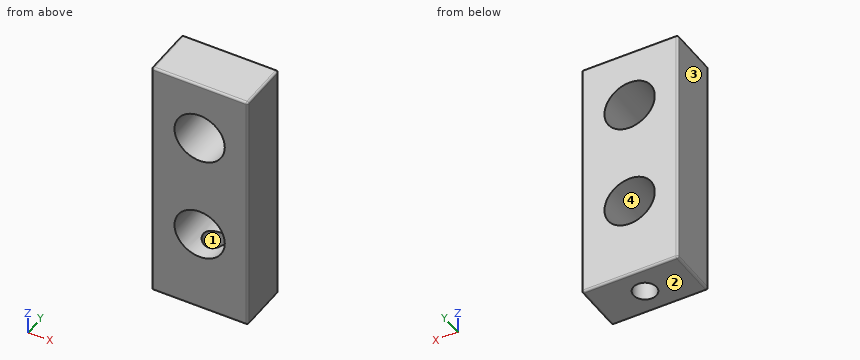
```python
from build123d import *

# Parameters (mm, degrees)
F0_W     = 58.42
F0_H     = 149.86
F0_R     = 15.24
F1_DEPTH = 31.75
F2_R     = 6.985
F3_DEPTH = 46.99
F4_R     = 1.27


with BuildPart() as f1:
    # F0 (on Front) → F1 (new body)
    with BuildSketch(Plane.XZ):
        with Locations((-19.275324, 10.416049)):
            Rectangle(F0_W, F0_H)
        with Locations((-19.275324, -14.983951)):
            Circle(F0_R, mode=Mode.SUBTRACT)
        with Locations((-19.275324, 49.786049)):
            Circle(F0_R, mode=Mode.SUBTRACT)
    extrude(amount=F1_DEPTH)

    # F2 (on face) → F3 (cut)
    with BuildSketch(Plane(origin=(0, 0, -64.513951), x_dir=(1, 0, 0), z_dir=(0, 0, -1))):
        with Locations((-19.275324, 15.875)):
            Circle(F2_R)
    extrude(amount=-F3_DEPTH, mode=Mode.SUBTRACT)

    # F4
    f4_edges = [f1.edges().sort_by_distance(p)[0] for p in [
        (-48.485324, -31.75, 10.416049),
        (9.934676, -31.75, 10.416049),
        (-19.275324, -31.75, -64.513951),
        (-19.275324, -31.75, 85.346049),
        (-48.485324, -15.875, -64.513951),
        (9.934676, -15.875, -64.513951),
        (-48.485324, 0, 10.416049),
        (9.934676, -15.875, 85.346049),
        (9.934676, 0, 10.416049),
        (-19.275324, 0, -64.513951),
        (-19.275324, 0, 85.346049),
        (-48.485324, -15.875, 85.346049),
    ]]
    fillet(f4_edges, radius=F4_R)


solid = f1.part
```
Work out the finished part from the listing and answer in its coordinate system (mm). Face numbers are marked on the shaded views. Give positions to 0.01 mm unless a question says otherwise; leave off trailing zeros. Loops run counter-clockwise (first coordinate to the right, second up) from the corner with the lowest first, then second, coordinate; pieces in that order, holes last. Notation, with made-up numbers: (-15.75, -27.5) - (-3.75, -27.5) arc R31 cw to (-3.75, 6.5) - close; hole circle Ø3 at (80, 51.25). An arc over 180 degrees is marked (long way). Use CSV: the item, a comma, the result in double quotes. Start each with the question number.
(1) Determine the mould class of the marked faces 1, 2, 3 and 4 for opening direction X: released by +X, released by -X, zero draft, split by the parting line, or undercut.
(2) Find section B-B, the plane x = -15.5. Determine the outline of the cut face in (y, z).
(3) Find section D-D, the plane x = -23. Determine the outline of the cut face in (y, z).
(4) Find section C-C, the plane y = -25.5. Determine the outline of the cut face in (x, z), plus the area to 3 significant figures.
(5) Find the intervals of material crossed by L1, parallel to Z at x = -10.5, y = -30; L2, parallel to Z at x = -6, y = -7.5; L3, parallel to X at y = -6.5, z = 63.5, in increasing order.
(6) Find section A-A, the plane z = -20. Determine the outline of the cut face in (x, y), plus the area to 3 significant figures.
Results found:
1,face 1,"undercut"
1,face 2,"zero draft"
1,face 3,"released by -X"
1,face 4,"undercut"
2,outline,"(-31.75, -63.24) arc R1.27 ccw to (-30.48, -64.51) - (-21.75, -64.51) - (-21.75, -29.75) - (-31.75, -29.75) - close; (-31.75, -0.22) - (0, -0.22) - (0, 35.02) - (-31.75, 35.02) - close; (-31.75, 64.55) - (0, 64.55) - (0, 84.08) arc R1.27 ccw to (-1.27, 85.35) - (-30.48, 85.35) arc R1.27 ccw to (-31.75, 84.08) - close; (-10, -64.51) - (-1.27, -64.51) arc R1.27 ccw to (0, -63.24) - (0, -29.75) - (-10, -29.75) - close"
3,outline,"(-31.75, -63.24) arc R1.27 ccw to (-30.48, -64.51) - (-21.78, -64.51) - (-21.78, -29.76) - (-31.75, -29.76) - close; (-31.75, -0.21) - (0, -0.21) - (0, 35.01) - (-31.75, 35.01) - close; (-31.75, 64.56) - (0, 64.56) - (0, 84.08) arc R1.27 ccw to (-1.27, 85.35) - (-30.48, 85.35) arc R1.27 ccw to (-31.75, 84.08) - close; (-9.97, -64.51) - (-1.27, -64.51) arc R1.27 ccw to (0, -63.24) - (0, -29.76) - (-9.97, -29.76) - close"
4,outline,"(-48.49, -63.24) arc R1.27 ccw to (-47.22, -64.51) - (8.66, -64.51) arc R1.27 ccw to (9.93, -63.24) - (9.93, 84.08) arc R1.27 ccw to (8.66, 85.35) - (-47.22, 85.35) arc R1.27 ccw to (-48.49, 84.08) - close; hole circle Ø30.48 at (-19.28, -14.98); hole circle Ø30.48 at (-19.28, 49.79)"
4,area,"7,290 mm^2"
5,L1,"-64.51 to -27.44, -2.52 to 37.33, 62.25 to 85.35"
5,L2,"-64.51 to -22.47, -7.5 to 42.3, 57.27 to 85.35"
5,L3,"-48.49 to -25.92, -12.63 to 9.93"
6,outline,"(-48.49, -30.48) arc R1.27 ccw to (-47.22, -31.75) - (-33.67, -31.75) - (-33.67, 0) - (-47.22, 0) arc R1.27 ccw to (-48.49, -1.27) - close; (-4.88, -31.75) - (8.66, -31.75) arc R1.27 ccw to (9.93, -30.48) - (9.93, -1.27) arc R1.27 ccw to (8.66, 0) - (-4.88, 0) - close"
6,area,"940 mm^2"
